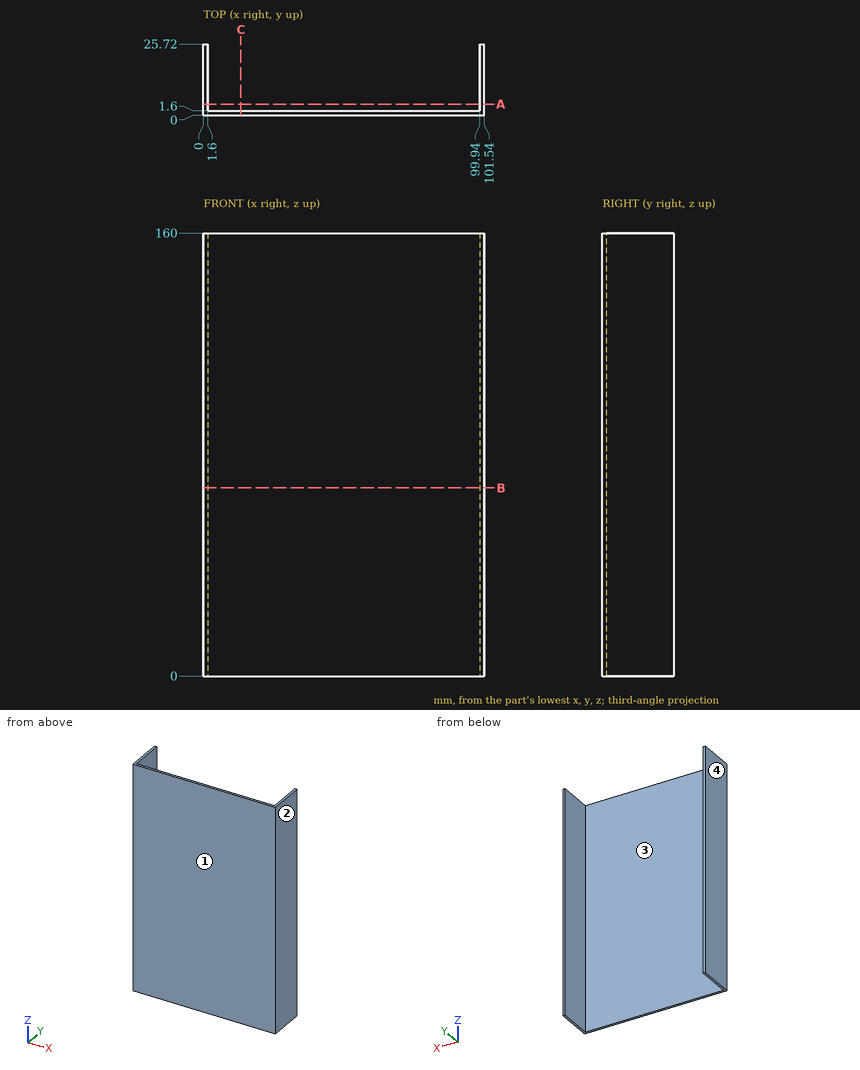
Part print with two shaded views. Sizes in mm from the minimum x, y, z corner. Coordinates: 2 decimals unless noted, no trailing zeros. Order: outer loops, then holes, each group sorted by start corner. A loop starts at its lowest first (then second) coordinate and runs counter-clockwise, first axis right, second up. Notation, with made-up numbers: (87.5, 69.25) - (114.5, 69.25) arc R25 cw to (114.5, 101.25) - close; hole circle Ø1 at (49.5, 52). An arc over 180 degrees is marked (long way). Write item = value, one per line. Start each with the question number.
1) Saw through at A-A on y = 4. Write the cut outline in (x, z), then the cut area to 3 significant figures.
2) Two-plate mould, pull along X, no slides. Class the marked faces 1, 2, 3 and 4: pulls with the +X half, pulls with the -X half, needs draft (parallel to the pull), parting line crosses it, or undercut.
3) Flat gauge pin, fed straight in: pin 1 Ø6 at (x, z) = (70, 79) entering from +Y. Where does the tip first touch, or does it go through?
4) Wall check: line 1 along X through (y, z) = (24.25, 77); line 2 along Y through (x, z) = (44, 17). Give the ranges that are in metal, low to high. Write a range as from..to.
5) Saw through at B-B on z = 68. Write the cut outline in (x, y).
6) Saw through at C-C on x = 13.5. Write the cut outline in (y, z), then the cut area to 3 significant figures.
From the geometry:
q1.outline = (0, 0) - (1.6, 0) - (1.6, 160) - (0, 160) - close; (99.94, 0) - (101.54, 0) - (101.54, 160) - (99.94, 160) - close
q1.area = 512 mm^2
q2.face_1 = needs draft
q2.face_2 = pulls with the +X half
q2.face_3 = undercut
q2.face_4 = pulls with the -X half
q3.pin_1 = 1.6
q4.line_1 = 0..1.6, 99.94..101.54
q4.line_2 = 0..1.6
q5.outline = (0, 0) - (101.54, 0) - (101.54, 25.72) - (99.94, 25.72) - (99.94, 1.6) - (1.6, 1.6) - (1.6, 25.72) - (0, 25.72) - close
q6.outline = (0, 0) - (1.6, 0) - (1.6, 160) - (0, 160) - close
q6.area = 256 mm^2
